Verification items for the finished model (mm, model axes). Face numbers are marked on the shaded views. A direction names the side the tool comes from. Give positions to 0.01 mm unless a question says otherwise; leave off trailing zeros. Loops run counter-clockwise (first coordinate to the right, second up) from the corner with the lowest first, then second, coordinate; pieces in that order, holes last. Notation, with made-up numbers: (0, -21.75) - (25, -21.75) arc R23 cw to (25, 17.25) - close; hole circle Ø8 at (45, 70). An arc over 180 degrees is marked (long way). Answer in a Markdown table with one row per item.
```python
from build123d import *

# Parameters (mm, degrees)
SKETCH1_R           = 1.6
BOSS_EXTRUDE1_DEPTH = 1.2
SKETCH2_W           = 29
SKETCH2_H           = 1.2
BOSS_EXTRUDE2_DEPTH = 15
CUT_EXTRUDE1_DEPTH  = 45.913027063
FILLET1_R           = 1.2
FILLET2_R           = 1.2
FILLET3_R           = 2


with BuildPart() as part:
    # Sketch1 → Boss-Extrude1 (new body)
    with BuildSketch(Plane(origin=(0, 0, 0), x_dir=(0, 0, -1), z_dir=(1, 0, 0))):
        with BuildLine():
            Line((-7.5, 0), (7.5, 0))
            Line((7.5, 0), (10.108191381, 0))
            ThreePointArc((10.108191381, 0), (10.773771613, -0.253673694), (11.101671453, -0.88599409))
            Line((11.101671453, -0.88599409), (14.493480072, -30.44318348))
            ThreePointArc((14.493480072, -30.44318348), (14.498368687, -30.500093294), (14.5, -30.55718939))
            Line((14.5, -30.55718939), (14.5, -40.5))
            Line((14.5, -40.5), (-14.5, -40.5))
            Line((-14.5, -40.5), (-14.5, -30.556102861))
            ThreePointArc((-14.5, -30.556102861), (-14.498368572, -30.499004746), (-14.493479611, -30.442092935))
            Line((-14.493479611, -30.442092935), (-11.101674621, -0.885990074))
            ThreePointArc((-11.101674621, -0.885990074), (-10.773773734, -0.253672349), (-10.10819501, 0))
            Line((-10.10819501, 0), (-7.5, 0))
        make_face()
        with Locations((-7.5, -3.5)):
            Circle(SKETCH1_R, mode=Mode.SUBTRACT)
        with Locations(Location((7.5, -3.5, 0), (0, 0, 180))):
            Circle(SKETCH1_R, mode=Mode.SUBTRACT)
        with BuildLine():
            ThreePointArc((6.769643375, -33.224825582), (9.311234852, -31.868958813), (11.721023336, -30.290674494))
            ThreePointArc((11.721023336, -30.290674494), (12.081311767, -28.067489873), (9.858127146, -27.707201442))
            ThreePointArc((9.858127146, -27.707201442), (7.687475006, -29.128864072), (5.398099397, -30.350180849))
            ThreePointArc((5.398099397, -30.350180849), (4.64654902, -32.473275205), (6.769643375, -33.224825582))
        make_face(mode=Mode.SUBTRACT)
        with BuildLine():
            ThreePointArc((-6.769643375, -33.224825582), (-9.311234852, -31.868958813), (-11.721023336, -30.290674494))
            ThreePointArc((-11.721023336, -30.290674494), (-12.081311767, -28.067489873), (-9.858127146, -27.707201442))
            ThreePointArc((-9.858127146, -27.707201442), (-7.687475006, -29.128864072), (-5.398099397, -30.350180849))
            ThreePointArc((-5.398099397, -30.350180849), (-4.64654902, -32.473275205), (-6.769643375, -33.224825582))
        make_face(mode=Mode.SUBTRACT)
    extrude(amount=BOSS_EXTRUDE1_DEPTH)

    # Sketch2 → Boss-Extrude2 (add)
    with BuildSketch(Plane(origin=(1.2, 0, 0), x_dir=(0, 0, -1), z_dir=(1, 0, 0))):
        with Locations((0, -39.9)):
            Rectangle(SKETCH2_W, SKETCH2_H)
    extrude(amount=BOSS_EXTRUDE2_DEPTH)

    # Sketch3 → Cut-Extrude1 (cut, through all)
    with BuildSketch(Plane(origin=(0, -39.3, 0), x_dir=(1, 0, 0), z_dir=(0, 1, 0))):
        with BuildLine():
            Line((8.25, -3.5), (8.25, 10.5))
            ThreePointArc((8.25, 10.5), (10, 12.25), (11.75, 10.5))
            Line((11.75, 10.5), (11.75, -3.5))
            ThreePointArc((11.75, -3.5), (10, -5.25), (8.25, -3.5))
        make_face()
        with BuildLine():
            ThreePointArc((7.23117506, -12.08087557), (10, -12.24726258), (12.76882494, -12.08087557))
            ThreePointArc((12.76882494, -12.08087557), (14.296662597, -10.133900456), (12.349687483, -8.606062799))
            ThreePointArc((12.349687483, -8.606062799), (10, -8.74726258), (7.650312517, -8.606062799))
            ThreePointArc((7.650312517, -8.606062799), (5.703337403, -10.133900456), (7.23117506, -12.08087557))
        make_face()
    extrude(amount=-CUT_EXTRUDE1_DEPTH, mode=Mode.SUBTRACT)

    # Fillet1
    fillet1_edges = [part.edges().sort_by_distance(p)[0] for p in [
        (1.2, -39.3, 0),
    ]]
    fillet(fillet1_edges, radius=FILLET1_R)

    # Fillet2
    fillet2_edges = [part.edges().sort_by_distance(p)[0] for p in [
        (0, -40.5, 0),
    ]]
    fillet(fillet2_edges, radius=FILLET2_R)

    # Fillet3
    fillet3_edges = [part.edges().sort_by_distance(p)[0] for p in [
        (16.2, -39.9, 14.5),
        (16.2, -39.9, -14.5),
    ]]
    fillet(fillet3_edges, radius=FILLET3_R)


solid = part.part
```
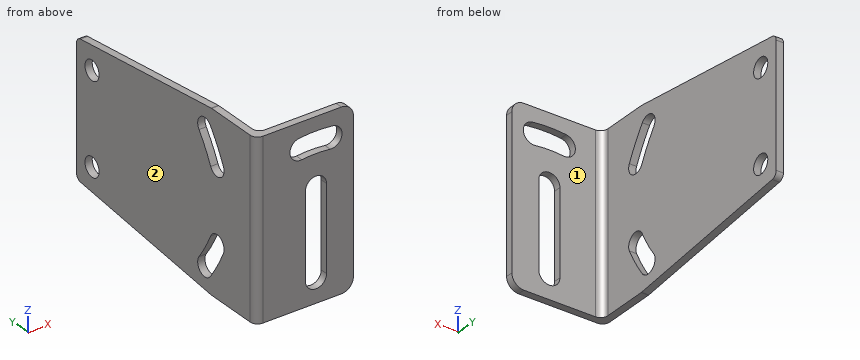
Q1. Go/stop test with flat-tipped pins: P1, Ø7, axis at x = 6.5, z = 3.5, coming from the +Y side; P2, Ø5, axis at y = -3.5, z = 7.5, coming from the +X side; P3, Ø8, axis at x = 3, y = -18.5, coming from the -Z side. Record where each tip stops, or that it passes through.
Completed:
| item | result |
|---|---|
| P1 | y = -39.3 |
| P2 | x = 1.2 |
| P3 | z = -13.53 |
Q2. Sectioned sample at D-D (z = 7.5). Record the cut outline in (x, y).
Completed:
| item | result |
|---|---|
| outline | (0, -39.3) arc R1.2 ccw to (1.2, -40.5) - (16.2, -40.5) - (16.2, -39.3) - (2.4, -39.3) arc R1.2 cw to (1.2, -38.1) - (1.2, -32.86) - (0, -32.86) - close; (0, -29.24) - (1.2, -29.24) - (1.2, -5.1) - (0, -5.1) - close; (0, -1.9) - (1.2, -1.9) - (1.2, 0) - (0, 0) - close |
Q3. Tool access check on the marked faces 1 and 2. Record the directions out of +Z, -Z, +X, -X, +Y, -Y that give a thin tool (end or side, any length) a straight path to the whole face; none if there is none.
Completed:
| item | result |
|---|---|
| face 1 | +Z, -Z, +X, +Y |
| face 2 | +Z, -Z, -X, +Y, -Y |
Q4. Sectioned sample at B-B (x = 10). Record the cut outline in (y, z).
Completed:
| item | result |
|---|---|
| outline | (-40.5, -14.5) - (-39.3, -14.5) - (-39.3, -12.25) - (-40.5, -12.25) - close; (-40.5, 5.25) - (-39.3, 5.25) - (-39.3, 8.75) - (-40.5, 8.75) - close; (-40.5, 12.25) - (-39.3, 12.25) - (-39.3, 14.5) - (-40.5, 14.5) - close |
Q5. Thickness scan on line 1 (Y direction, x = 0.8, z = 7.5); line 2 (Y direction, x = 0.4, z = 7.5); line 3 (Y direction, x = 11.25, z = 6.5). Record the ranges inside material, lowest first.
Completed:
| item | result |
|---|---|
| line 1 | -40.43 to -32.86, -29.24 to -5.1, -1.9 to 0 |
| line 2 | -40.19 to -32.86, -29.24 to -5.1, -1.9 to 0 |
| line 3 | -40.5 to -39.3 |
Q6. Sectioned sample at C-C (y = -3.5). Record the cut outline in (x, z), and give its area (3 significant figures).
Completed:
| item | result |
|---|---|
| outline | (0, -11.4) - (1.2, -11.4) - (1.2, -9.1) - (0, -9.1) - close; (0, -5.9) - (1.2, -5.9) - (1.2, 5.9) - (0, 5.9) - close; (0, 9.1) - (1.2, 9.1) - (1.2, 11.4) - (0, 11.4) - close |
| area | 19.7 mm^2 |
Q7. Sectioned sample at A-A (z = -0.75). Record the cut outline in (x, y).
Completed:
| item | result |
|---|---|
| outline | (0, -39.3) arc R1.2 ccw to (1.2, -40.5) - (8.25, -40.5) - (8.25, -39.3) - (2.4, -39.3) arc R1.2 cw to (1.2, -38.1) - (1.2, 0) - (0, 0) - close; (11.75, -40.5) - (16.2, -40.5) - (16.2, -39.3) - (11.75, -39.3) - close |
